Here's how the part is built. I have some questions about the finished solid (model axes, mm). A direction names the side the tool comes from. Coordinates: 2 decimals unless noted, no trailing zeros. Order: outer loops, then holes, each group sorted by start corner. A loop starts at its lowest first (then second) coordinate and runs counter-clockwise, first axis right, second up. Notation, with made-up numbers: M -7,-13.75 L 35,-13.75 A18 ccw 35,13.25 Z; hole C -36.5,65.5 d7. An arc over 180 degrees is marked long. One line per question, with ' | ' between items. Start each with the question number.
```python
from build123d import *

# Parameters (mm, degrees)
F0_W     = 10
F0_H     = 15
F0_R     = 2
F1_DEPTH = 2


with BuildPart() as f1:
    # F0 (on Top) → F1 (new body)
    with BuildSketch(Plane.XY):
        Polygon((-33.75, -15), (33.75, -15), (33.75, -7.5), (33.75, 7.5), (33.75, 15), (-33.75, 15), (-33.75, 7.5), (-33.75, -7.5), align=None)
        with Locations((-38.75, 0)):
            Rectangle(F0_W, F0_H)
        with Locations((-38.75, 0)):
            Circle(F0_R, mode=Mode.SUBTRACT)
        with Locations((38.75, 0)):
            Rectangle(F0_W, F0_H)
        with Locations((38.75, 0)):
            Circle(F0_R, mode=Mode.SUBTRACT)
    extrude(amount=F1_DEPTH)


solid = f1.part
```
1. I need wall thicknesses on line 1 (Y direction, x = 38.75, z = 0.5); line 2 (X direction, y = 1.25, z = 1.75); line 3 (Y direction, x = -34.5, z = 1.95). Which ranges of each line are inside material? Lowest first, please.
2. Imagine slicing it at B-B (x = -38.75). List the corners of the cut face in (y, z) for me, then the cut area to 3 significant figures.
3. We'd pull the mould along Y, two halves only. Please class faces 4 (the face through (-40.748, 0.088, 0.986)), 5 (the face through (-1, 0, 0)), 6 (the face through (39, 7.5, 1)), 7 (the face through (36.752, 0.088, 0.986)): released by +Y, released by -Y, zero draft, split by the parting line, or undercut.
4. Imagine slicing it at D-D (y = -13). List the corners of the cut face in (x, z) for me, then the cut area to 3 significant figures.
5. Imagine slicing it at A-A (z = 1.4). List the corners of the cut face in (x, y) for me, then the cut area to 3 significant figures.
6. Imagine slicing it at C-C (y = 0). List the corners of the cut face in (x, z) for me.
7. Which directions (+Z, -Z, +X, -X, +Y, -Y) give clear straight access to the entire face, cutting with the end or side of a thin tool? Please do faces 1 (the face through (39, -7.5, 1)), 2 (the face through (-33.75, -11, 1)), 3 (the face through (-33.75, 11, 1)).
8. Will these pins go through, and if not, where does the flat tip stop? pin 1 (3.5 mm diameter, centred on x = 38.75, y = 0, fed in from +Z); pin 2 (1 mm diameter, centred on x = 38, z = 1, fed in from +Y); pin 3 (1 mm diameter, centred on x = 39.5, z = 1, fed in from -Y); pin 4 (0.6 mm diameter, centred on y = -10, z = 0.5, fed in from -X).
Entries:
1) line 1: -7.5 to -2, 2 to 7.5 | line 2: -43.75 to -40.31, -37.19 to 37.19, 40.31 to 43.75 | line 3: -7.5 to 7.5
2) outline: M -7.5,0 L -2,0 L -2,2 L -7.5,2 Z; M 2,0 L 7.5,0 L 7.5,2 L 2,2 Z | area: 22.0 mm²
3) face 4: undercut | face 5: zero draft | face 6: released by +Y | face 7: undercut
4) outline: M -33.75,0 L 33.75,0 L 33.75,2 L -33.75,2 Z | area: 135 mm²
5) outline: M -43.75,-7.5 L -33.75,-7.5 L -33.75,-15 L 33.75,-15 L 33.75,-7.5 L 43.75,-7.5 L 43.75,7.5 L 33.75,7.5 L 33.75,15 L -33.75,15 L -33.75,7.5 L -43.75,7.5 Z; hole C -38.75,0 d4; hole C 38.75,0 d4 | area: 2,300 mm²
6) outline: M -43.75,0 L -40.75,0 L -40.75,2 L -43.75,2 Z; M -36.75,0 L 36.75,0 L 36.75,2 L -36.75,2 Z; M 40.75,0 L 43.75,0 L 43.75,2 L 40.75,2 Z
7) face 1: +Z, -Z, +X, -Y | face 2: +Z, -Z, -X, -Y | face 3: +Z, -Z, -X, +Y
8) pin 1: through | pin 2: y = 7.5 | pin 3: y = -7.5 | pin 4: x = -33.75
